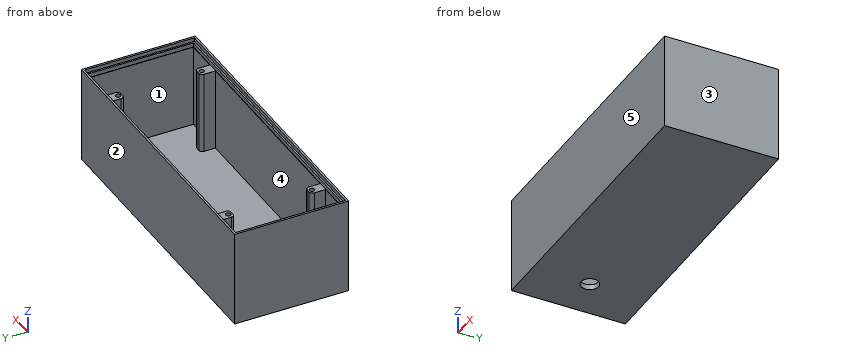
```python
from build123d import *

# Parameters (mm, degrees)
SKETCH_W        = 166.8
SKETCH_H        = 64.8
PAD_DEPTH       = 54.6
SKETCH001_W     = 164.4
SKETCH001_H     = 62.4
POCKET_DEPTH    = 2.2
SKETCH002_W     = 162.4
SKETCH002_H     = 60.4
POCKET001_DEPTH = 2.4
SKETCH003_R     = 1.417537
SKETCH003_R_2   = 1.403016
SKETCH003_R_3   = 1.376417
SKETCH003_R_4   = 1.428442
POCKET002_DEPTH = 10
POCKET003_DEPTH = 47
SKETCH005_R     = 4.970408
POCKET004_DEPTH = 3
FILLET_R        = 2


with BuildPart() as part:
    # Sketch → Pad (new body)
    with BuildSketch(Plane.XY):
        Rectangle(SKETCH_W, SKETCH_H)
    extrude(amount=PAD_DEPTH)

    # Sketch001 (on Face6 of Pad) → Pocket (cut)
    with BuildSketch(Plane.XY.offset(54.6)):
        Rectangle(SKETCH001_W, SKETCH001_H)
    extrude(amount=-POCKET_DEPTH, mode=Mode.SUBTRACT)

    # Sketch002 (on Face11 of Pocket) → Pocket001 (cut)
    with BuildSketch(Plane.XY.offset(52.4)):
        Rectangle(SKETCH002_W, SKETCH002_H)
    extrude(amount=-POCKET001_DEPTH, mode=Mode.SUBTRACT)

    # Sketch003 (on Face16 of Pocket001) → Pocket002 (cut)
    with BuildSketch(Plane.XY.offset(50)):
        with Locations((-60, 23.8)):
            Circle(SKETCH003_R)
        with Locations((-60, -23.8)):
            Circle(SKETCH003_R_2)
        with Locations((60, -23.8)):
            Circle(SKETCH003_R_3)
        with Locations((60, 23.8)):
            Circle(SKETCH003_R_4)
    extrude(amount=-POCKET002_DEPTH, mode=Mode.SUBTRACT)

    # Sketch004 (on Face16 of Pocket002) → Pocket003 (cut)
    with BuildSketch(Plane.XY.offset(50)):
        Polygon((-81, -30), (-81, 30), (-63, 30), (-63, 21.6), (-57, 21.6), (-57, 30), (57, 30), (57, 21.6), (63, 21.6), (63, 30), (81, 30), (81, -30), (63, -30), (63, -21.6), (57, -21.6), (57, -30), (-57, -30), (-57, -21.6), (-63, -21.6), (-63, -30), align=None)
    extrude(amount=-POCKET003_DEPTH, mode=Mode.SUBTRACT)

    # Sketch005 (on Face44 of Pocket003) → Pocket004 (cut)
    with BuildSketch(Plane.XY.offset(3)):
        with Locations((-60.009918, 0)):
            Circle(SKETCH005_R)
    extrude(amount=-POCKET004_DEPTH, mode=Mode.SUBTRACT)

    # Fillet
    fillet_edges = [part.edges().sort_by_distance(p)[0] for p in [
        (-63, 21.6, 26.5),
        (-57, 21.6, 26.5),
        (57, 21.6, 26.5),
        (63, 21.6, 26.5),
        (63, -21.6, 26.5),
        (-57, -21.6, 26.5),
        (57, -21.6, 26.5),
        (-63, -21.6, 26.5),
    ]]
    fillet(fillet_edges, radius=FILLET_R)


solid = part.part
```
Verification items for the finished model (mm, model axes). Face numbers are marked on the shaded views. A direction names the side the tool comes from. Give positions to 0.01 mm unless a question says otherwise; leave off trailing zeros. Order: outer loops, then holes, each group sorted by start corner. A loop starts at its lowest first (then second) coordinate and runs counter-clockwise, first axis right, second up. Notation, with made-up numbers: (41.25, 1.25) -> (45.25, 1.25) arc R22 ccw to (45.25, 13.25) -> close; hole circle Ø8 at (54, 21). An arc over 180 degrees is marked (long way). Use a Markdown table: item, result.
1) Depth check by flat-ended pin: pin 1 Ø2.5 at (x, y) = (60, -23.8) entering from +Z; pin 2 Ø10 at (x, y) = (-25, 0.5) entering from +Z; pin 3 Ø3 at (x, y) = (-59.5, -24) entering from +Z. Enter the tip coordinate at first touch or a pass-through.
Results:
| item | result |
|---|---|
| pin 1 | z = 40 |
| pin 2 | z = 3 |
| pin 3 | z = 50 |
2) Tool access check on the marked faces 4 and 5. Record the directions out of +Z, -Z, +X, -X, +Y, -Y that give a thin tool (end or side, any length) a straight path to the whole face; none if there is none.
Results:
| item | result |
|---|---|
| face 4 | +Z |
| face 5 | +Z, -Z, +X, -X, -Y |
3) Mould release check, pull along Y, two halves, no side actions. Record for the marked faces 1, 2 and 3: pulls with the +Y half, pulls with the -Y half, needs draft (parallel to the pull), parting line crosses it, or undercut.
Results:
| item | result |
|---|---|
| face 1 | undercut |
| face 2 | pulls with the +Y half |
| face 3 | needs draft |
4) Section check A-A, the plane y = 0. Record the boundary of the cut face in (x, z).
Results:
| item | result |
|---|---|
| outline | (-83.4, 0) -> (-64.98, 0) -> (-64.98, 3) -> (-81, 3) -> (-81, 50) -> (-81.2, 50) -> (-81.2, 52.4) -> (-82.2, 52.4) -> (-82.2, 54.6) -> (-83.4, 54.6) -> close; (-55.04, 0) -> (83.4, 0) -> (83.4, 54.6) -> (82.2, 54.6) -> (82.2, 52.4) -> (81.2, 52.4) -> (81.2, 50) -> (81, 50) -> (81, 3) -> (-55.04, 3) -> close |
5) Material ranges on probe 1 along X at (y, z) = (25.5, 35); probe 2 along Y at (x, z) = (56.5, 14); probe 3 along X at (y, z) = (-6.5, 38), recorded low to high.
Results:
| item | result |
|---|---|
| probe 1 | -83.4 to -81, -63 to -57, 57 to 63, 81 to 83.4 |
| probe 2 | -32.4 to -30, 30 to 32.4 |
| probe 3 | -83.4 to -81, 81 to 83.4 |
6) Section check C-C, the plane y = 17. Record the boundary of the cut face in (x, z).
Results:
| item | result |
|---|---|
| outline | (-83.4, 0) -> (83.4, 0) -> (83.4, 54.6) -> (82.2, 54.6) -> (82.2, 52.4) -> (81.2, 52.4) -> (81.2, 50) -> (81, 50) -> (81, 3) -> (-81, 3) -> (-81, 50) -> (-81.2, 50) -> (-81.2, 52.4) -> (-82.2, 52.4) -> (-82.2, 54.6) -> (-83.4, 54.6) -> close |
7) Section check D-D, the plane x = 37. Record the boundary of the cut face in (y, z), then the cut area to 3 significant figures.
Results:
| item | result |
|---|---|
| outline | (-32.4, 0) -> (32.4, 0) -> (32.4, 54.6) -> (31.2, 54.6) -> (31.2, 52.4) -> (30.2, 52.4) -> (30.2, 50) -> (30, 50) -> (30, 3) -> (-30, 3) -> (-30, 50) -> (-30.2, 50) -> (-30.2, 52.4) -> (-31.2, 52.4) -> (-31.2, 54.6) -> (-32.4, 54.6) -> close |
| area | 436 mm² |
